Design review of the part shown in the three views and the two pictorial views. Dimensions are in mm from the part's minimum x, y and z. Give positions to 0.01 mm unless a question says otherwise; leave off trailing zeros. Loops run counter-clockwise (first coordinate to the right, second up) from the corner with the lowest first, then second, coordinate; pieces in that order, holes last. Notation, with made-up numbers: (52.25, -20) - (72.25, -20) arc R23 cw to (72.25, 16) - close; hole circle Ø3 at (58, 4). An arc over 180 degrees is marked (long way). Answer in a Markdown table with one row per item.
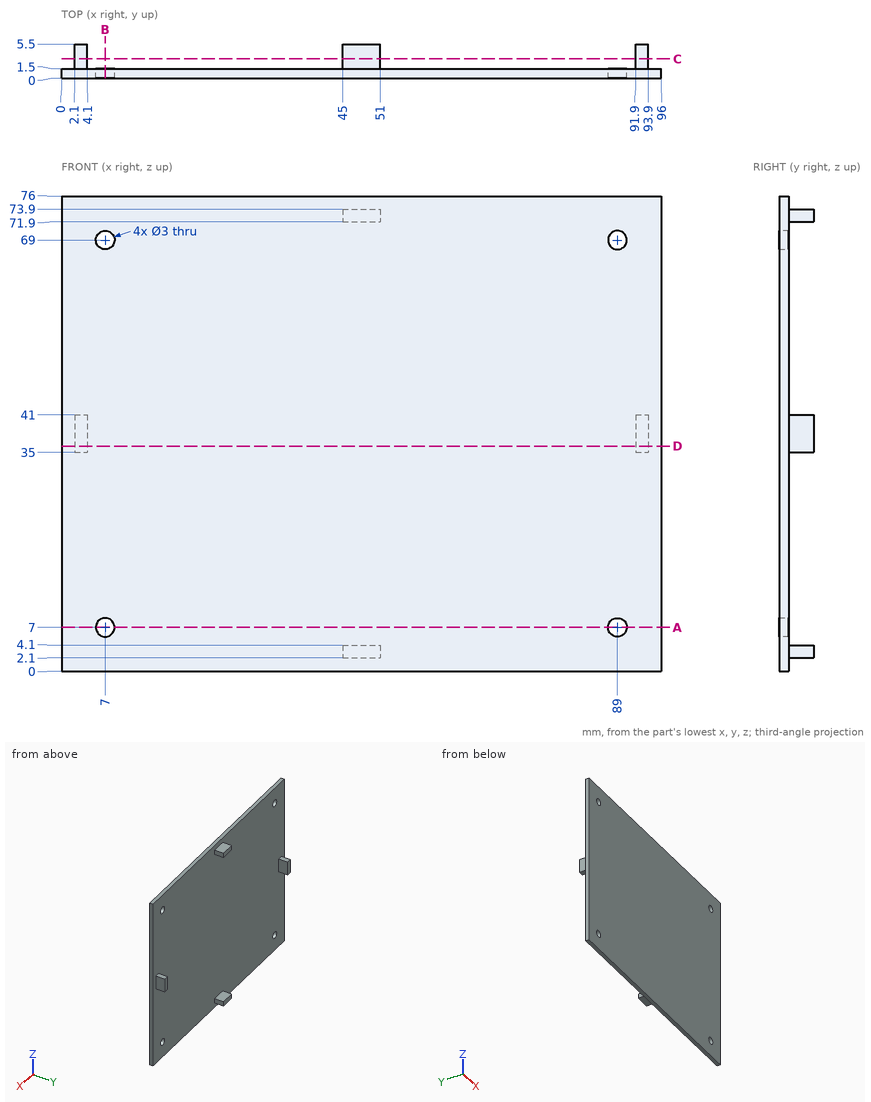
1. Clearance check with flat-ended pins moving along their axes: pin 1 (1 mm diameter, centred on x = 3, y = 4, fed in from -Z); pin 2 (1.2 mm diameter, centred on x = 47.5, y = 4, fed in from -Z); pin 3 (1 mm diameter, centred on x = 49.5, y = 3, fed in from +Z). State where each tip first meets the part, or that it passes through.
Values:
| item | result |
|---|---|
| pin 1 | stops at z = 35 |
| pin 2 | stops at z = 2.1 |
| pin 3 | stops at z = 73.9 |
2. We need section B-B, the plane x = 7. Give the boundary of the cut face in (y, z), and give its area (3 significant figures).
Values:
| item | result |
|---|---|
| outline | (0, 0) - (1.5, 0) - (1.5, 5.5) - (0, 5.5) - close; (0, 8.5) - (1.5, 8.5) - (1.5, 67.5) - (0, 67.5) - close; (0, 70.5) - (1.5, 70.5) - (1.5, 76) - (0, 76) - close |
| area | 105 mm^2 |
3. Wall thickness on line 1 (Z direction, x = 89, y = 0.65); line 2 (X direction, y = 0.4, z = 7); line 3 (Z direction, x = 48, y = 2.8): over which ranges is each line inside the solid? List them lowest first. Write a range as [from, to].
Values:
| item | result |
|---|---|
| line 1 | z = [0, 5.5], [8.5, 67.5], [70.5, 76] |
| line 2 | x = [0, 5.5], [8.5, 87.5], [90.5, 96] |
| line 3 | z = [2.1, 4.1], [71.9, 73.9] |
4. We need section A-A, the plane z = 7. Give the boundary of the cut face in (x, y), and give its area (3 significant figures).
Values:
| item | result |
|---|---|
| outline | (0, 0) - (5.5, 0) - (5.5, 1.5) - (0, 1.5) - close; (8.5, 0) - (87.5, 0) - (87.5, 1.5) - (8.5, 1.5) - close; (90.5, 0) - (96, 0) - (96, 1.5) - (90.5, 1.5) - close |
| area | 135 mm^2 |
5. We need section D-D, the plane z = 36. Give the boundary of the cut face in (x, y), and give its area (3 significant figures).
Values:
| item | result |
|---|---|
| outline | (0, 0) - (96, 0) - (96, 1.5) - (93.9, 1.5) - (93.9, 5.5) - (91.9, 5.5) - (91.9, 1.5) - (4.1, 1.5) - (4.1, 5.5) - (2.1, 5.5) - (2.1, 1.5) - (0, 1.5) - close |
| area | 160 mm^2 |
6. We need section C-C, the plane y = 3.1. Give the boundary of the cut face in (x, z), and give its area (3 significant figures).
Values:
| item | result |
|---|---|
| outline | (2.1, 35) - (4.1, 35) - (4.1, 41) - (2.1, 41) - close; (45, 2.1) - (51, 2.1) - (51, 4.1) - (45, 4.1) - close; (45, 71.9) - (51, 71.9) - (51, 73.9) - (45, 73.9) - close; (91.9, 35) - (93.9, 35) - (93.9, 41) - (91.9, 41) - close |
| area | 48.0 mm^2 |
